Autodesk Inventor part; units mm, degrees
ref_plane "YZ Plane" through (0, 0, 0) normal (1, 0, 0) x (0, 1, 0)
ref_plane "XZ Plane" through (0, 0, 0) normal (0, 1, 0) x (-1, 0, 0)
ref_plane "XY Plane" through (0, 0, 0) normal (0, 0, 1) x (1, 0, 0)
sketch "Sketch1" plane through (0, 0, 0) normal (0, 0, 1) x (1, 0, 0)
  line L0 (0, 0) -> (20, 0)
  line L1 (20, 0) -> (20, 20)
  line L2 (20, 20) -> (0, 20)
  line L3 (0, 20) -> (0, 0)
  dimension "d0" = 20
  dimension "d1" = 20
extrude "Extrusion1" add sketch "Sketch1" along normal blind 152.5
sketch "Sketch2" plane through (0, 20, 0) normal (0, 1, 0) x (1, 0, 0)
  line L0 (0, -152.5) -> (20, -152.5)
  line L1 (0, 0) -> (0, -152.5)
  line L2 (0, -80) -> (8, -80)
  line L3 (8, -80) -> (8, -67)
  line L4 (8, -67) -> (0, -67)
  line L5 (0, -67) -> (0, -80)
  dimension "d4" = 13
  dimension "d5" = 72.5
  dimension "d6" = 8
extrude "Extrusion2" cut sketch "Sketch2" against normal blind 20
sketch "Sketch3" plane through (0, 20, 0) normal (0, 1, 0) x (1, 0, 0)
  line L0 (0, -80) -> (0, -152.5)
  line L1 (0, -152.5) -> (20, -152.5)
  line L2 (20, 0) -> (20, -152.5)
  line L3 (0, -137.5) -> (20, -137.5)
  dimension "d9" = 15
extrude "Extrusion3" cut sketch "Sketch3" against normal blind 10
chamfer "Chamfer1" distance 7 angle 45 1 edges at (20, 5, 152.5)
sketch "Sketch4" plane through (0, 20, 0) normal (0, 1, 0) x (1, 0, 0)
  line L0 (0, -137.5) -> (10, -137.5)
  line L1 (10, -137.5) -> (10, -112.5)
  line L2 (10, -112.5) -> (0, -112.5)
  line L3 (0, -112.5) -> (0, -137.5)
  dimension "d15" = 10
  dimension "d16" = 25
extrude "Extrusion4" cut sketch "Sketch4" against normal blind 10
chamfer "Chamfer2" distance 10 angle 45 1 edges at (10, 10, 125)
sketch "Sketch5" plane through (0, 0, 0) normal (0, -1, 0) x (1, 0, 0)
  line L0 (0, 80) -> (0, 152.5)
  line L1 (20, 137.5) -> (0, 137.5)
  point P0 (10, 145)
  dimension "d22" = 10
  dimension "d23" = 7.5
hole "Hole1" at (10, 0, 145) direction (0, 1, 0) diameter 6.5 depth 10 tip angle 118 counterbore diameter 10 counterbore depth 7
sketch "Sketch6" plane through (20, 0, 0) normal (1, 0, 0) x (0, 0, -1)
  line L0 (0, 0) -> (-145.5, 0)
  line L1 (-80, 20) -> (-80, 0)
  line L2 (-67, 20) -> (-67, 0)
  line L3 (-152.5, 10) -> (-152.5, 0)
  point P0 (-73.5, 10)
  dimension "d31" = 79
  dimension "d32" = 10
hole "Hole2" at (20, 10, 73.5) direction (-1, 0, 0) diameter 6.5 depth 13 tip angle 118 counterbore diameter 10 counterbore depth 7
sketch "Sketch7" plane through (0, 0, 0) normal (-1, 0, 0) x (0, 0, 1)
  line L0 (0, 20) -> (67, 20)
  line L1 (0, 20) -> (0, 0)
  line L2 (42, 20) -> (22, 20)
  line L3 (22, 20) -> (22, 15)
  line L4 (22, 15) -> (42, 15)
  line L5 (42, 15) -> (42, 20)
  dimension "d40" = 20
  dimension "d41" = 22
  dimension "d42" = 5
extrude "Extrusion5" cut sketch "Sketch7" against normal blind 20
sketch "Sketch8" plane through (0, 0, 0) normal (0, -1, 0) x (1, 0, 0)
  line L0 (20, 0) -> (20, 145.5)
  line L1 (0, 22) -> (20, 22)
  line L2 (0, 42) -> (20, 42)
  point P0 (10, 32)
  dimension "d45" = 10
  dimension "d46" = 10
hole "Hole3" at (10, 0, 32) direction (0, 1, 0) diameter 6.5 depth 15 tip angle 118 counterbore diameter 10 counterbore depth 7
sketch "Sketch9" plane through (0, 0, 0) normal (-1, 0, 0) x (0, 0, 1)
  line L0 (0, 0) -> (67, 0)
  line L1 (42, 15) -> (22, 15)
  line L2 (27, 7) -> (27, 0)
  line L3 (27, 7) -> (37, 7)
  line L4 (37, 7) -> (37, 0)
  line L5 (35.25, 15) -> (35.25, 7)
  line L6 (28.75, 15) -> (28.75, 7)
  line L7 (32, 15) -> (32, 0)
  point P0 (39.5, 10)
  point P1 (24.5, 10)
  dimension "d54" = 15
  dimension "d56" = 7.5
  dimension "d57" = 10
hole "Hole4" at (0, 10, 39.5) at (0, 10, 24.5) direction (1, 0, 0) diameter 3.2 depth 12 tip angle 118
sketch "Sketch10" plane through (0, 0, 0) normal (0, 0, -1) x (-1, 0, 0)
  line L0 (-20, 20) -> (0, 20)
  line L1 (-20, 0) -> (-20, 20)
  point P0 (-13, 10)
  dimension "d65" = 7
  dimension "d66" = 10
hole "Hole5" at (13, 10, 0) direction (0, 0, 1) diameter 4.917 depth 8 tip angle 118
chamfer "Chamfer3" distance 0.5 angle 45 1 edges at (13, 7.5415, 0)
sketch "Sketch11" plane through (0, 0, 0) normal (-1, 0, 0) x (0, 0, 1)
  line L0 (0, 20) -> (22, 20)
  line L1 (0, 20) -> (0, 0)
  point P0 (6.5, 10)
  dimension "d77" = 10
  dimension "d78" = 6.5
hole "Hole6" at (0, 10, 6.5) direction (1, 0, 0) diameter 4.917 depth 8 tip angle 118
chamfer "Chamfer4" distance 0.5 angle 45 1 edges at (0, 10, 4.0415)
properties part number "CHASSI ESQUERDO(37)" material "Carbon Steel"
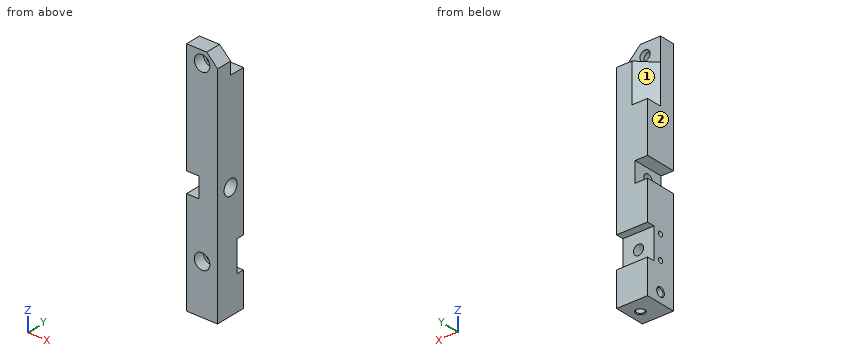
Here's how the part is built. I have some questions about the finished solid (model axes, mm). Face numbers are marked on the shaded views. A direction names the side the tool comes from. Give positions to 0.01 mm unless a question says otherwise; leave off trailing zeros. Order: outer loops, then holes, each group sorted by start corner. A loop starts at its lowest first (then second) coordinate and runs counter-clockwise, first axis right, second up. Notation, with made-up numbers: (44.5, 68.25) -> (102.5, 68.25) arc R26 ccw to (102.5, 95.25) -> close; hole circle Ø6 at (-37.5, 33.25). An arc over 180 degrees is marked (long way). Use a Markdown table: item, result. Add a question column.
Item 1: For the marked faces 1 and 2, which set-ups out of +Z, -Z, +X, -X, +Y, -Y let a thin tool reach every point of the face, with its end or its side?
Item 2: I need wall thicknesses on line 1 (Z direction, x = 10, y = 5.5); line 2 (Y direction, x = 3, z = 39.5); line 3 (Y direction, x = 4.75, z = 6.5). Which ranges of each line are inside material? Lowest first, please.
Item 3: Imagine slicing it at A-A on z = 73.5. Please give me the cut outline in (x, y), plus the area to 4 significant figures.
Item 4: Will these pins go through, and if not, where does the flat tip stop? pin 1 (3 mm diameter, centred on y = 15.5, z = 112.5, fed in from -X); pin 2 (3 mm diameter, centred on x = 8, z = 33, fed in from -Y); pin 3 (9 mm diameter, centred on y = 10, z = 73.5, fed in from -X); pin 4 (4 mm diameter, centred on x = 7.5, z = 29, fed in from +Y).
Item 5: Imagine slicing it at C-C on x = 18.5. Please give me the cut outline in (y, z).
Item 6: Imagine slicing it at B-B on y = 2.5. Please give me the cut outline in (x, z).
Data:
| question | item | result |
|---|---|---|
| 1 | face 1 | +Z, -X, +Y |
| 1 | face 2 | +Z, -Z, -X, +Y, -Y |
| 2 | line 1 | z = 0 to 27, 37 to 140, 150 to 152.5 |
| 2 | line 2 | y = 0 to 8.4, 11.6 to 15 |
| 2 | line 3 | y = 0 to 7.54, 12.46 to 20 |
| 3 | outline | (8, 0) -> (20, 0) -> (20, 5) -> (13, 5) -> (13, 6.75) -> (8, 6.75) -> close; (8, 13.25) -> (13, 13.25) -> (13, 15) -> (20, 15) -> (20, 20) -> (8, 20) -> close |
| 3 | area | 137.5 mm² |
| 4 | pin 1 | stops at x = 0 |
| 4 | pin 2 | stops at y = 7 |
| 4 | pin 3 | stops at x = 8 |
| 4 | pin 4 | stops at y = 15 |
| 5 | outline | (0, 0) -> (20, 0) -> (20, 22) -> (15, 22) -> (15, 42) -> (20, 42) -> (20, 137.5) -> (10, 137.5) -> (10, 147) -> (0, 147) -> close; hole circle Ø10 at (10, 73.5) |
| 6 | outline | (0, 0) -> (20, 0) -> (20, 145.5) -> (13, 152.5) -> (0, 152.5) -> (0, 80) -> (8, 80) -> (8, 67) -> (0, 67) -> close; hole circle Ø10 at (10, 32); hole circle Ø10 at (10, 145) |
